```python
from build123d import *

# Parameters (mm, degrees)
SKETCH_1_W      = 25
SKETCH_1_H      = 10
EXTRUDE_1_DEPTH = 15
SKETCH_2_R      = 2
EXTRUDE_2_DEPTH = 3
SKETCH_3_W      = 2
SKETCH_3_H      = 10
EXTRUDE_3_DEPTH = 3.5
SKETCH_4_W      = 2
SKETCH_4_H      = 10
EXTRUDE_4_DEPTH = 3.5
EXTRUDE_START   = 2
SKETCH_7_R      = 2.5
EXTRUDE_5_DEPTH = 0.5


with BuildPart() as part:
    # 스케치1 → 보스-돌출1 (new body)
    with BuildSketch(Plane.XY):
        Rectangle(SKETCH_1_W, SKETCH_1_H)
    extrude(amount=EXTRUDE_1_DEPTH)

    # 스케치2 → 보스-돌출2 (add)
    with BuildSketch(Plane.XY.offset(15)):
        with Locations((-7.5, 0)):
            Circle(SKETCH_2_R)
    extrude(amount=EXTRUDE_2_DEPTH)

    # 스케치3 → 보스-돌출3 (add)
    with BuildSketch(Plane(origin=(12.5, 0, 0), x_dir=(0, 0, -1), z_dir=(1, 0, 0))):
        with Locations((-11, 0)):
            Rectangle(SKETCH_3_W, SKETCH_3_H)
    extrude(amount=EXTRUDE_3_DEPTH)

    # 스케치4 → 보스-돌출4 (add)
    with BuildSketch(Plane.ZY.offset(12.5)):
        with Locations((11, 0)):
            Rectangle(SKETCH_4_W, SKETCH_4_H)
    extrude(amount=EXTRUDE_4_DEPTH)

    # 스케치7 → 보스-돌출5 (add)
    with BuildSketch(Plane.XY.offset(15).offset(EXTRUDE_START)):
        with Locations((-7.5, 0)):
            Circle(SKETCH_7_R)
    extrude(amount=EXTRUDE_5_DEPTH)


solid = part.part
```
Work out the finished part from the listing and answer in its coordinate system (mm). A direction names the side the tool comes from. Round coordinates to 2 decimals unless told otherwise and drop trailing zeros. Loops run counter-clockwise (first coordinate to the right, second up) from the corner with the lowest first, then second, coordinate; pieces in that order, holes last.
(1) Find the intervals of material crossed by L1, parallel to Z at x = -2.5, y = -4.5; L2, parallel to X at y = 4, z = 5.25; L3, parallel to Y at x = -7.5, z = 16.5, in increasing order.
Computed values:
L1: z = 0 to 15
L2: x = -12.5 to 12.5
L3: y = -2 to 2
(2) Each of these flat-tipped pins is pushed along its axis until it touches: P1, Ø3, axis at y = 0, z = 4, coming from the -X side; P2, Ø1, axis at x = -4.5, y = 2, coming from the +Z side; P3, Ø6, axis at y = -3, z = 6, coming from the +X side. Where does it stop, or does it pass through?
Computed values:
P1: stops at x = -12.5
P2: stops at z = 15
P3: stops at x = 12.5
(3) For faces 1 (the cylindrical face through (-9.498, 0.088, 15.986)), 2 (the flat face through (-14, 0, 12)), 3 (the flat face through (14, 0, 10)), 4 (the flat face through (-12.5, 0, 5)), 5 (the cylindrical face through (-9.498, 0.088, 17.746)), determine the directions among +Z, -Z, +X, -X, +Y, -Y from which every point of the face is accessible in a straight line to the end or side of a thin tool.
Computed values:
face 1: none
face 2: +Z, -X, +Y, -Y
face 3: -Z, +X, +Y, -Y
face 4: -Z, -X, +Y, -Y
face 5: +Z
(4) The part is cut by section D-D, the plane y = 4. Give the vertices of the cut face in (x, z), and give its area (3 significant figures).
Computed values:
outline: (-16, 10) - (-12.5, 10) - (-12.5, 0) - (12.5, 0) - (12.5, 10) - (16, 10) - (16, 12) - (12.5, 12) - (12.5, 15) - (-12.5, 15) - (-12.5, 12) - (-16, 12) - close
area: 389 mm2
(5) The part is cut by section B-B, the plane x = -7.5. Give the vertices of the cut face in (y, z).
Computed values:
outline: (-5, 0) - (5, 0) - (5, 15) - (2, 15) - (2, 17) - (2.5, 17) - (2.5, 17.5) - (2, 17.5) - (2, 18) - (-2, 18) - (-2, 17.5) - (-2.5, 17.5) - (-2.5, 17) - (-2, 17) - (-2, 15) - (-5, 15) - close
(6) The part is cut by section C-C, the plane z = 12.5. Give the vertices of the cut face in (x, y), and give its area (3 significant figures).
Computed values:
outline: (-12.5, -5) - (12.5, -5) - (12.5, 5) - (-12.5, 5) - close
area: 250 mm2
(7) The part is cut by section A-A, the plane y = 0. Give the vertices of the cut face in (x, z).
Computed values:
outline: (-16, 10) - (-12.5, 10) - (-12.5, 0) - (12.5, 0) - (12.5, 10) - (16, 10) - (16, 12) - (12.5, 12) - (12.5, 15) - (-5.5, 15) - (-5.5, 17) - (-5, 17) - (-5, 17.5) - (-5.5, 17.5) - (-5.5, 18) - (-9.5, 18) - (-9.5, 17.5) - (-10, 17.5) - (-10, 17) - (-9.5, 17) - (-9.5, 15) - (-12.5, 15) - (-12.5, 12) - (-16, 12) - close
